```python
from build123d import *

# Parameters (mm, degrees)
SKETCH1_R           = 15
BOSS_EXTRUDE1_DEPTH = 145
BOSS_EXTRUDE2_START = 50
SKETCH2_R           = 5
BOSS_EXTRUDE2_DEPTH = 20
SHELL1_START        = -125
SHELL1_DEPTH        = 250
SKETCH4_W           = 520
SKETCH4_H           = 290
BOSS_EXTRUDE3_DEPTH = 20
FILLET1_R           = 20


# Read off the part's stored shape, not the designer's step: Shell1
with BuildPart() as part:
    # Sketch1 → Boss-Extrude1 (new, symmetric)
    with BuildSketch(Plane.XY):
        with BuildLine():
            Line((0, 0), (0, 120))
            Line((0, 120), (228.31744945, 120))
            ThreePointArc((228.31744945, 120), (239.69359838, 121.311364411), (250.473016236, 125.176670579))
            Line((250.473016236, 125.176670579), (366.167012988, 182.362651739))
            ThreePointArc((366.167012988, 182.362651739), (389.803653925, 187.517381697), (413.093568272, 180.972007347))
            Line((413.093568272, 180.972007347), (520, 120))
            Line((520, 120), (520, 0))
            Line((520, 0), (0, 0))
        make_face()
        with Locations((388.322579774, 140)):
            Circle(SKETCH1_R, mode=Mode.SUBTRACT)
    extrude(amount=BOSS_EXTRUDE1_DEPTH, both=True)

    # Sketch2 → Boss-Extrude2 (add)
    with BuildSketch(Plane.XY.offset(BOSS_EXTRUDE2_START)):
        with BuildLine():
            Line((0, 120), (0, 204))
            ThreePointArc((0, 204), (12.346331353, 222.47759065), (34.142135624, 218.142135624))
            Line((34.142135624, 218.142135624), (122.284271247, 130))
            Line((122.284271247, 130), (260.23118156, 130))
            Line((260.23118156, 130), (250.473016236, 125.176670579))
            ThreePointArc((250.473016236, 125.176670579), (239.69359838, 121.311364411), (228.31744945, 120))
            Line((228.31744945, 120), (0, 120))
        make_face()
        with Locations((20, 204)):
            Circle(SKETCH2_R, mode=Mode.SUBTRACT)
        with Locations((45, 179)):
            Circle(SKETCH2_R, mode=Mode.SUBTRACT)
    boss_extrude2 = extrude(amount=-BOSS_EXTRUDE2_DEPTH)

    # Mirror1: Boss-Extrude2 across plane
    add(boss_extrude2.mirror(Plane.XY))

    # Shell1 outline → Shell1 (cut)
    with BuildSketch(Plane.XY.offset(SHELL1_START)):
        with BuildLine():
            Line((356.937260838, 155.490698991), (259.33524295, 107.247338811))
            ThreePointArc((259.33524295, 107.247338811), (244.244057952, 101.835910175), (228.31744945, 100))
            Line((228.31744945, 100), (20, 100))
            Line((20, 100), (20, 0))
            Line((20, 0), (500, 0))
            Line((500, 0), (500, 108.382476706))
            Line((500, 108.382476706), (420.526102167, 153.708871052))
            ThreePointArc((420.526102167, 153.708871052), (387.342226815, 105.013732579), (356.937260838, 155.490698991))
        make_face()
    extrude(amount=SHELL1_DEPTH, mode=Mode.SUBTRACT)

    # Sketch4 → Boss-Extrude3 (add)
    # profile 1 of 2: a face of its own
    with BuildSketch(Plane.XZ):
        Polygon((540, 165), (0, 165), (0, 145), (520, 145), (520, -145), (0, -145), (0, -165), (540, -165), align=None)
    # profile 2 of 2: a face of its own
    with BuildSketch(Plane.XZ):
        with Locations((260, 0)):
            Rectangle(SKETCH4_W, SKETCH4_H)
        Polygon((20, 125), (228.31744945, 125), (259.33524295, 125), (353.322579774, 125), (356.937260838, 125), (420.526102167, 125), (423.322579774, 125), (500, 125), (500, -125), (423.322579774, -125), (420.526102167, -125), (356.937260838, -125), (353.322579774, -125), (259.33524295, -125), (228.31744945, -125), (20, -125), align=None, mode=Mode.SUBTRACT)
    extrude(amount=-BOSS_EXTRUDE3_DEPTH)

    # Fillet1
    fillet1_edges = [part.edges().sort_by_distance(p)[0] for p in [
        (389.803653925, 187.517381697, -145),
        (466.546784136, 150.486003673, -145),
        (466.546784136, 150.486003673, 145),
        (389.803653925, 187.517381697, 145),
        (308.320014612, 153.769661159, 145),
        (239.69359838, 121.311364411, 145),
        (114.158724725, 120, 145),
        (114.158724725, 120, -145),
        (239.69359838, 121.311364411, -145),
        (308.320014612, 153.769661159, -145),
    ]]
    fillet(fillet1_edges, radius=FILLET1_R)


solid = part.part
```
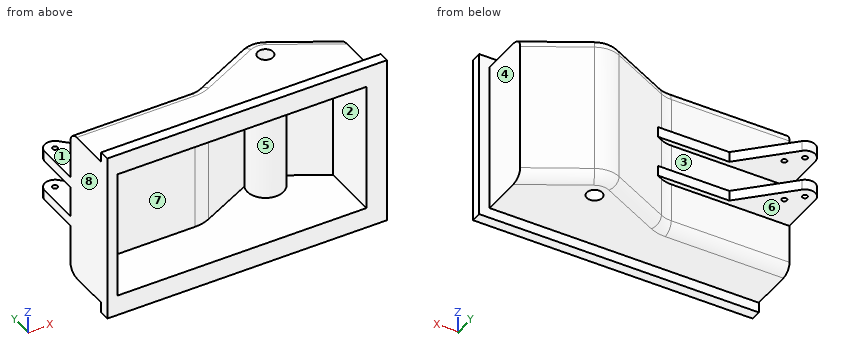
Verification items for the finished model (mm, model axes). Face numbers are marked on the shaded views. A direction names the side the tool comes from. Round coordinates to 2 decimals unless told otherwise and drop trailing zeros. Write each loop counter-clockwise with the first axis right and the second up, starting at its lowest first coordinate (ties: lowest second). Pieces come first, ordered by that corner, then holes. Notation, with made-up numbers: (77, 39.25) - (122, 39.25) arc R30 ccw to (122, 67.25) - close; hole circle Ø5 at (-27.75, 66). An arc over 180 degrees is marked (long way). Answer as a JSON object with one key per item and string values. Group by question number.
Q1. Section check B-B, the plane z = 119. Enter the section's corners in (x, y), plus the area to 3 significant figures.
Q2. Mould release check, pull along X, two halves, no side actions. Record for the marked faces 6, 7 and 8: released by +X, released by -X, zero draft, split by the parting line, or undercut.
Q3. Tool access check on the marked faces 1, 2, 3, 4 and 5. Record the directions out of +Z, -Z, +X, -X, +Y, -Y that give a thin tool (end or side, any length) a straight path to the whole face; none if there is none.
Q4. Section check C-C, the plane y = 140. Give the number of separate pieces and of enclosed holes in the cut face, plus the area to 3 significant figures.
Q5. Go/stop test with flat-tipped pins: pin 1 Ø6 at (y, z) = (154.5, -57.5) entering from -X; pin 2 Ø8 at (y, z) = (152.5, 63.5) entering from -X; pin 3 Ø5 at (x, z) = (216.5, -125) entering from +Y; pin 4 Ø3 at (y, z) = (104.5, 30) entering from -X. Record where each tip stops, or that it passes through.
Q6. Thickness scan on line 1 (Z direction, x = 474.5, y = 50.5); line 2 (X direction, y = 147, z = 105); line 3 (X direction, y = 128, z = -108.5). Record the ranges inside material, lowest first.
Q7. Section check A-A, the plane y = 69. Enter the section's corners in (x, z).
Found:
{
 "1": {"outline": "(0, 0) - (20, 0) - (20, 100) - (228.32, 100) arc R70 ccw to (259.34, 107.25) - (356.94, 155.49) arc R35 ccw (long way) to (420.53, 153.71) - (500, 108.38) - (500, 0) - (540, 0) - (540, 20) - (520, 20) - (520, 120) - (413.09, 180.97) arc R50 ccw to (366.17, 182.36) - (250.47, 125.18) arc R50 cw to (228.32, 120) - (0, 120) - close; hole circle Ø30 at (388.32, 140)", "area": "18,200 mm^2"},
 "2": {"face 6": "zero draft", "face 7": "undercut", "face 8": "released by -X"},
 "3": {"face 1": "+Z, -X, +Y", "face 2": "-Y", "face 3": "-X, +Y", "face 4": "+Z, -Z, +X, +Y", "face 5": "none"},
 "4": {"separate pieces": "4", "enclosed holes": "2", "area": "42,100 mm^2"},
 "5": {"pin 1": "stops at x = 303.73", "pin 2": "stops at x = 297.66", "pin 3": "stops at y = 120", "pin 4": "stops at x = 0"},
 "6": {"line 1": "z = -145 to -125, 125 to 145", "line 2": "x = 294.62 to 339.76, 354.03 to 375.06, 401.59 to 422.62, 432.29 to 472.66", "line 3": "x = 256.18 to 301.32, 355.44 to 379.32, 397.32 to 421.2, 465.6 to 505.97"},
 "7": {"outline": "(0, -145) - (520, -145) - (520, 145) - (0, 145) - close; hole (20, -125) - (500, -125) - (500, 125) - (20, 125) - close"}
}
